from build123d import *

# Parameters (mm, degrees)
SZKIC1_W                                   = 736.8
SZKIC1_H                                   = 167.4
DODANIE_WYCI_GNI_CIE1_DEPTH                = 10
SZKIC2_W                                   = 729.8
SZKIC2_H                                   = 160.4
SZKIC2_W_2                                 = 723.8
SZKIC2_H_2                                 = 154.4
WYCI_CIE_WYCI_GNI_CIE_CIENKA_CIANKA1_DEPTH = 3
SZKIC3_W                                   = 713.8
SZKIC3_H                                   = 144.4
WYTNIJ_WYCI_GNI_CIE1_DEPTH                 = 5
ZAOKR_GLENIE1_R                            = 3
SZKIC4_R                                   = 4
SZKIC4_R_2                                 = 2
DODANIE_WYCI_GNI_CIE2_DEPTH                = 10
SZKIC4_3_R                                 = 2
WYTNIJ_WYCI_GNI_CIE2_DEPTH                 = 10


with BuildPart() as part:
    # Szkic1 → Dodanie-wyci_gni_cie1 (new body)
    with BuildSketch(Plane(origin=(0, 0, 0), x_dir=(1, 0, 0), z_dir=(0, 1, 0))):
        with Locations((35.673743017, 109.761452514)):
            Rectangle(SZKIC1_W, SZKIC1_H)
    extrude(amount=DODANIE_WYCI_GNI_CIE1_DEPTH)

    # Szkic2 → Wyci_cie-wyci_gni_cie-cienka _cianka1 (cut)
    with BuildSketch(Plane.XZ):
        with Locations((35.673743017, -109.761452514)):
            Rectangle(SZKIC2_W, SZKIC2_H)
        with Locations((35.673743017, -109.761452514)):
            Rectangle(SZKIC2_W_2, SZKIC2_H_2, mode=Mode.SUBTRACT)
    extrude(amount=-WYCI_CIE_WYCI_GNI_CIE_CIENKA_CIANKA1_DEPTH, mode=Mode.SUBTRACT)

    # Szkic3 → Wytnij-wyci_gni_cie1 (cut)
    with BuildSketch(Plane.XZ):
        with Locations((35.673743017, -109.761452514)):
            Rectangle(SZKIC3_W, SZKIC3_H)
    extrude(amount=-WYTNIJ_WYCI_GNI_CIE1_DEPTH, mode=Mode.SUBTRACT)

    # Zaokr_glenie1
    zaokr_glenie1_edges = [part.edges().sort_by_distance(p)[0] for p in [
        (-329.226256983, 1.5, -189.961452514),
        (-329.226256983, 1.5, -29.561452514),
        (400.573743017, 1.5, -29.561452514),
        (400.573743017, 1.5, -189.961452514),
        (-326.226256983, 1.5, -32.561452514),
        (397.573743017, 1.5, -32.561452514),
        (397.573743017, 1.5, -186.961452514),
        (-321.226256983, 2.5, -181.961452514),
    ]]
    fillet(zaokr_glenie1_edges, radius=ZAOKR_GLENIE1_R)

    # Szkic4 → Dodanie-wyci_gni_cie2 (add)
    with BuildSketch(Plane.XZ):
        with Locations((-313.726256983, -173.061452514)):
            Circle(SZKIC4_R)
        with Locations((-313.726256983, -173.061452514)):
            Circle(SZKIC4_R_2, mode=Mode.SUBTRACT)
        with Locations((385.073743017, -173.061452514)):
            Circle(SZKIC4_R)
        with Locations((385.073743017, -173.061452514)):
            Circle(SZKIC4_R_2, mode=Mode.SUBTRACT)
        with Locations((-313.726256983, -46.461452514)):
            Circle(SZKIC4_R)
        with Locations((385.073743017, -46.461452514)):
            Circle(SZKIC4_R)
    extrude(amount=-DODANIE_WYCI_GNI_CIE2_DEPTH)

    # Szkic4_3 → Wytnij-wyci_gni_cie2 (cut)
    with BuildSketch(Plane.XZ):
        with Locations((-313.726256983, -46.461452514)):
            Circle(SZKIC4_3_R)
        with Locations((-313.726256983, -173.061452514)):
            Circle(SZKIC4_3_R)
        with Locations((385.073743017, -173.061452514)):
            Circle(SZKIC4_3_R)
        with Locations((385.073743017, -46.461452514)):
            Circle(SZKIC4_3_R)
    extrude(amount=-WYTNIJ_WYCI_GNI_CIE2_DEPTH, mode=Mode.SUBTRACT)


solid = part.part
Could you check a few things on this model? Use its own coordinates, in mm. A direction names the side the tool comes from. Give positions to 0.01 mm unless a question says otherwise; leave off trailing zeros. Order: outer loops, then holes, each group sorted by start corner. A loop starts at its lowest first (then second) coordinate and runs counter-clockwise, first axis right, second up. Notation, with made-up numbers: (8, 8) -> (27, 8) arc R20 cw to (27, 41) -> close; hole circle Ø11 at (-21, 82.5). An arc over 180 degrees is marked (long way). Return JSON: item names as keys, results as strings.
1. I need wall thicknesses on line 1 (Z direction, x = 106.5, y = 2.25); line 2 (X direction, y = 1, z = -135); line 3 (Z direction, x = 224, y = 4.5). Which ranges of each line are inside material? Lowest first, please. Write a range as from..to.
Answer list:
{"line 1": "z = -193.46..-189.96, -186.96..-181.96, -37.56..-32.56, -29.56..-26.06", "line 2": "x = -332.73..-329.23, -326.23..-321.23, 392.57..397.57, 400.57..404.07", "line 3": "z = -193.46..-181.96, -37.56..-26.06"}
2. For pin 1 Ø3 at (x, z) = (-313.73, -173.06) entering from +Y; pin 2 Ø8 at (x, z) = (-139, -69.5) entering from -Y, each with a flat end and sliding along its axis, tell me the tip position at first contact or that it passes through.
Answer list:
{"pin 1": "passes through", "pin 2": "stops at y = 5"}
3. Imagine slicing it at A-A on x = 241. List the corners of the cut face in (y, z) for me.
Answer list:
{"outline": "(0, -193.46) -> (10, -193.46) -> (10, -26.06) -> (0, -26.06) -> (0, -29.56) -> (3, -29.56) -> (3, -32.56) -> (0, -32.56) -> (0, -37.56) -> (5, -37.56) -> (5, -181.96) -> (0, -181.96) -> (0, -186.96) -> (3, -186.96) -> (3, -189.96) -> (0, -189.96) -> close"}
4. Thinking about a two-plate mould opening in Z: for faces 1 (the flat face through (34, 0, -184)), 2 (the flat face through (34, 3, -32)), which applies, pulls with the +Z half, pulls with the -Z half, needs draft (parallel to the pull), parting line crosses it, or undercut?
Answer list:
{"face 1": "needs draft", "face 2": "undercut"}
5. On a 3-axis mill with a long thin cutter (end or side, diameter ignored), from which of +Z, -Z, +X, -X, +Y, -Y can I reach the whole of each face in a straight line? I mean faces 3 (the flat face through (31, 10, -111)), 4 (the flat face through (31, 5, -109)). Say none if no direction works.
Answer list:
{"face 3": "+Z, -Z, +X, -X, +Y", "face 4": "-Y"}
6. Imagine slicing it at B-B on z = -136.5. List the corners of the cut face in (x, y) for me.
Answer list:
{"outline": "(-332.73, 0) -> (-329.23, 0) -> (-329.23, 3) -> (-326.23, 3) -> (-326.23, 0) -> (-321.23, 0) -> (-321.23, 5) -> (392.57, 5) -> (392.57, 0) -> (397.57, 0) -> (397.57, 3) -> (400.57, 3) -> (400.57, 0) -> (404.07, 0) -> (404.07, 10) -> (-332.73, 10) -> close"}
